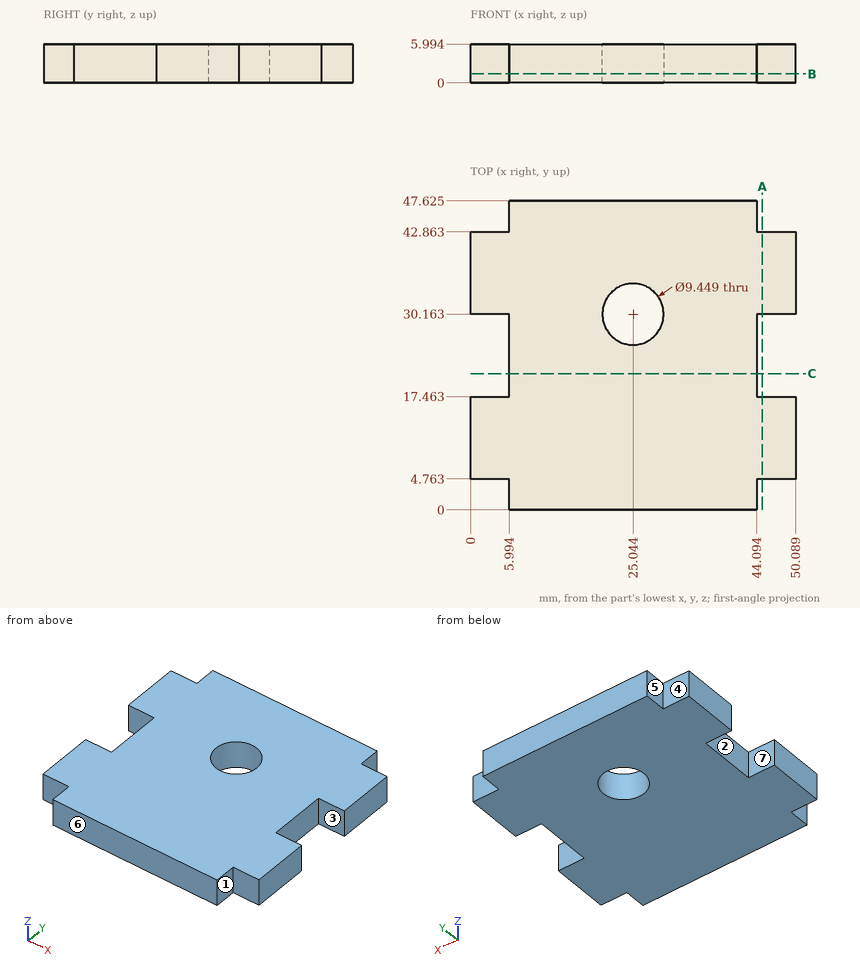
Print and shaded views of the part. All mm, measured from the part's lowest x, y and z. A direction names the side the tool comes from. Coordinates: 2 decimals unless noted, no trailing zeros. Order: outer loops, then holes, each group sorted by start corner. A loop starts at its lowest first (then second) coordinate and runs counter-clockwise, first axis right, second up. Notation, with made-up numbers: (34, -14.75) - (65, -14.75) arc R12 cw to (65, -6.75) - close; hole circle Ø2 at (51, -5). An arc over 180 degrees is marked (long way). Return JSON: item names as keys, results as strings. Group by question number.
Item 1: Cut at A-A (x = 45). List the corners of the cut face in (y, z) (1 decimal), plus the area to 3 significant figures.
Item 2: Cut at C-C (y = 21). List the corners of the cut face in (x, z) (1 decimal), plus the area to 3 significant figures.
Item 3: Pin check, flat tips, straight feed: pin 1 (3 mm diameter, centred on x = 3, z = 4.5, fed in from -Y); pin 2 (1 mm diameter, centred on x = 38, y = 35.5, fed in from -Z); pin 3 (2.5 mm diameter, centred on y = 45, z = 3, fed in from -X); pin 4 (3 mm diameter, centred on x = 46.5, z = 4.5, fed in from +Y). Stop position of each tip, or through.
Item 4: Pull direction Y, two halves, no side cores. Call the marked faces 5, 6 and 7: pulls with the +Y half, pulls with the -Y half, needs draft (parallel to the pull), parting line crosses it, or undercut.
Item 5: Which spindle directions (+Z, -Z, +X, -X, +Y, -Y) get a long thin tool onto all of the face, cutting with end or side? Do the marked faces 1, 2, 3 and 4. Say none if no direction does.
Item 6: Drill centre lines: probe 1 along Y at (x, z) = (3.5, 5.35); probe 2 along Y at (x, z) = (29, 2.15) (1 decimal); probe 3 along X at (y, z) = (45.5, 4.85) (1 decimal). Where is each one in solid material? Low to high. Write a range as from..to.
Item 7: Cut at B-B (z = 1.4). List the corners of the cut face in (x, y) (1 decimal), plus the area to 3 significant figures.
Check values:
{
 "1": {"outline": "(4.8, 0) - (17.5, 0) - (17.5, 6) - (4.8, 6) - close; (30.2, 0) - (42.9, 0) - (42.9, 6) - (30.2, 6) - close", "area": "152 mm2"},
 "2": {"outline": "(6, 0) - (44.1, 0) - (44.1, 6) - (6, 6) - close", "area": "228 mm2"},
 "3": {"pin 1": "stops at y = 4.76", "pin 2": "stops at z = 0", "pin 3": "stops at x = 5.99", "pin 4": "stops at y = 42.86"},
 "4": {"face 5": "needs draft", "face 6": "pulls with the -Y half", "face 7": "undercut"},
 "5": {"face 1": "+Z, -Z, +X, -Y", "face 2": "+Z, -Z, -X", "face 3": "+Z, -Z, +X", "face 4": "+Z, -Z, -X, +Y"},
 "6": {"probe 1": "y = 4.76..17.46, 30.16..42.86", "probe 2": "y = 0..27.6, 32.7..47.6", "probe 3": "x = 6..44.1"},
 "7": {"outline": "(0, 4.8) - (6, 4.8) - (6, 0) - (44.1, 0) - (44.1, 4.8) - (50.1, 4.8) - (50.1, 17.5) - (44.1, 17.5) - (44.1, 30.2) - (50.1, 30.2) - (50.1, 42.9) - (44.1, 42.9) - (44.1, 47.6) - (6, 47.6) - (6, 42.9) - (0, 42.9) - (0, 30.2) - (6, 30.2) - (6, 17.5) - (0, 17.5) - close; hole circle Ø9.4 at (25, 30.2)", "area": "2,050 mm2"}
}
